Work out the finished part from the listing and answer in its coordinate system (mm). Face numbers are marked on the shaded views. Give positions to 0.01 mm unless a question says otherwise; leave off trailing zeros. Loops run counter-clockwise (first coordinate to the right, second up) from the corner with the lowest first, then second, coordinate; pieces in that order, holes last. Notation, with made-up numbers: M 43.5,83 L 96.5,83 A25 ccw 96.5,111 Z; hole C 55.5,-37 d3. An arc over 180 degrees is marked long. Use a Markdown table: item, result.
```python
from build123d import *

# Parameters (mm, degrees)
F1_DEPTH       = 60
F3_D           = 5
F3_DEPTH       = 65
F3_CBORE_D     = 12
F3_CBORE_DEPTH = 25
F3_TIP         = 1.5021515476
F4_SIZE        = 1
F6_D           = 5
F6_DEPTH       = 23.5
F6_TIP         = 1.5021515476
F9_D           = 8
F9_ON_F7_D     = 8


with BuildPart() as f1:
    # F0 (on Top) → F1 (new body)
    with BuildSketch(Plane.XY):
        with BuildLine():
            Line((60, 35), (-60, 35))
            Line((-60, 35), (-60, -35))
            Line((-60, -35), (-16, -35))
            Line((-16, -35), (-16, -14.9749843554))
            ThreePointArc((-16, -14.9749843554), (-15, 25), (-14, -14.9749843554))
            Line((-14, -14.9749843554), (-14, -35))
            Line((-14, -35), (60, -35))
            Line((60, -35), (60, 35))
        make_face()
    extrude(amount=-F1_DEPTH)

    # F3
    with Locations(Plane(origin=(-60, 0, 0), x_dir=(0, -1, 0), z_dir=(-1, 0, 0))):
        with Locations((25, -45), (25, -15)):
            CounterBoreHole(F3_D / 2, F3_CBORE_D / 2, F3_CBORE_DEPTH, depth=F3_DEPTH)
            with Locations((0, 0, -(F3_DEPTH + F3_TIP / 2))):  # 118° drill point
                Cone(0, F3_D / 2, F3_TIP, mode=Mode.SUBTRACT)

    # F4
    f4_edges = [f1.edges().sort_by_distance(p)[0] for p in [
        (-60, -35, -30),
        (-60, 35, -30),
        (60, -35, -30),
        (60, 35, -30),
        (0, 35, -60),
        (-60, 0, -60),
        (-38, -35, -60),
        (23, -35, -60),
        (60, 0, -60),
        (-60, 0, 0),
        (-38, -35, 0),
        (23, -35, 0),
        (60, 0, 0),
        (0, 35, 0),
    ]]
    chamfer(f4_edges, length=F4_SIZE)

    # F6
    with Locations(Plane.YZ.offset(60)):
        with Locations((-22.5, -7.5), (22.5, -7.5), (22.5, -52.5), (-22.5, -52.5)):
            Hole(F6_D / 2, depth=F6_DEPTH)
            with Locations((0, 0, -(F6_DEPTH + F6_TIP / 2))):  # 118° drill point
                Cone(0, F6_D / 2, F6_TIP, mode=Mode.SUBTRACT)

    # F9 (through all)
    with Locations(Plane(origin=(0, 0, -60), x_dir=(1, 0, 0), z_dir=(0, 0, -1))):
        with Locations((15, -25), (15.2912072429, -10.0028269883), (15.5824144859, 4.9943460233), (15.8736217288, 19.991519035), (30.8736217288, 19.991519035), (30.5824144859, 4.9943460233), (30.2912072429, -10.0028269883), (30, -25)):
            Hole(F9_D / 2)

    # F9 on F7 (through all)
    with Locations(Plane(origin=(0, 0, -60), x_dir=(1, 0, 0), z_dir=(0, 0, -1))):
        with Locations((-50, -25), (-50, -10), (-50, 5)):
            Hole(F9_ON_F7_D / 2)


solid = f1.part
```
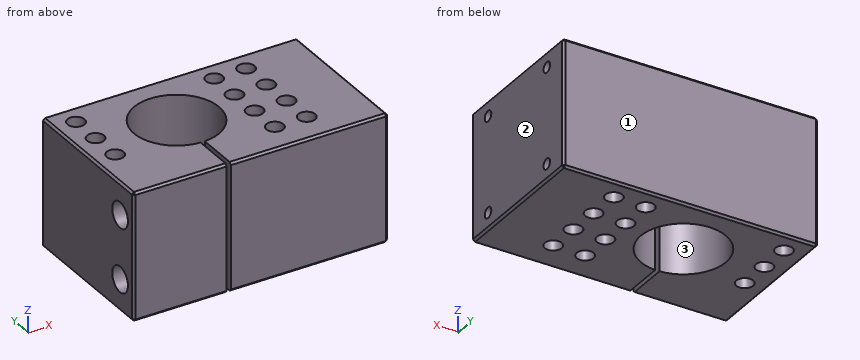
(1) The mould has two halves that part along Y. Classify the marked faces 1, 2 and 3: released by +Y, released by -Y, zero draft, split by the parting line, or undercut.
Entries:
| item | result |
|---|---|
| face 1 | released by +Y |
| face 2 | zero draft |
| face 3 | undercut |
(2) A cutting plane is placed at D-D (z = -34). Count the separate pieces of the cut face and the enclosed holes in it, and give its area (3 significant figures).
Entries:
| item | result |
|---|---|
| separate pieces | 1 |
| enclosed holes | 11 |
| area | 6,550 mm² |
(3) A cutting plane is placed at B-B (x = 40). Write down the section's boundary in (y, z).
Entries:
| item | result |
|---|---|
| outline | M -35,-59 L -34,-60 L 34,-60 L 35,-59 L 35,-1 L 34,0 L -34,0 L -35,-1 Z; hole C -22.5,-52.5 d5; hole C -22.5,-7.5 d5; hole C 22.5,-52.5 d5; hole C 22.5,-7.5 d5 |
(4) A cutting plane is placed at A-A (x = -50). Write down the section's boundary in (y, z).
Entries:
| item | result |
|---|---|
| outline | M -35,-59 L -34,-60 L -9,-60 L -9,0 L -34,0 L -35,-1 Z; M -1,-60 L 6,-60 L 6,0 L -1,0 Z; M 14,-60 L 21,-60 L 21,0 L 14,0 Z; M 29,-60 L 34,-60 L 35,-59 L 35,-1 L 34,0 L 29,0 Z; hole C -25,-45 d12; hole C -25,-15 d12 |
(5) Given P1, Ø6.5, axis at x = 15.29, y = 10, coming from the +Z side; P2, Ø9.5, axis at y = -24.5, z = -14, coming from the -X side, each flat-ended and moving along its own axis, determine where each tip first touches the part or whether it passes through.
Entries:
| item | result |
|---|---|
| P1 | passes through |
| P2 | stops at x = -35 |
(6) A cutting plane is placed at C-C (y = -12.5). Write down the section's boundary in (x, z), and give its area (3 significant figures).
Entries:
| item | result |
|---|---|
| outline | M -60,-59 L -59,-60 L -24.68,-60 L -24.68,0 L -59,0 L -60,-1 Z; M -5.32,-60 L 59,-60 L 60,-59 L 60,-1 L 59,0 L -5.32,0 Z |
| area | 6,040 mm² |
(7) Consider probe 1 along Y at (x, z) = (-50, -30); probe 2 along Y at (x, z) = (50.25, -52.5); probe 3 along Z at (x, y) = (50.75, -22.5). Determine where each line is inside the solid, lowest interval first. Write a range as [from, to].
Entries:
| item | result |
|---|---|
| probe 1 | y = [-35, -9], [-1, 6], [14, 21], [29, 35] |
| probe 2 | y = [-35, -25], [-20, 20], [25, 35] |
| probe 3 | z = [-60, -55], [-50, -10], [-5, 0] |
